Autodesk Inventor part; units mm, degrees
ref_plane "YZ Plane" through (0, 0, 0) normal (1, 0, 0) x (0, 1, 0)
ref_plane "XZ Plane" through (0, 0, 0) normal (0, 1, 0) x (-1, 0, 0)
ref_plane "XY Plane" through (0, 0, 0) normal (0, 0, 1) x (1, 0, 0)
sketch "Sketch1" plane through (0, 0, 0) normal (0, 0, 1) x (1, 0, 0)
  line L0 (-12.7, -12.7) -> (12.7, -12.7)
  line L1 (12.7, -12.7) -> (12.7, 12.7)
  line L2 (12.7, 12.7) -> (-12.7, 12.7)
  line L3 (-12.7, 12.7) -> (-12.7, -12.7)
  line L4 (-12.7, -12.7) -> (12.7, 12.7) construction
  line L5 (12.7, -12.7) -> (-12.7, 12.7) construction
  line L6 (-11.1125, -11.1125) -> (11.1125, -11.1125)
  line L7 (11.1125, -11.1125) -> (11.1125, 11.1125)
  line L8 (11.1125, 11.1125) -> (-11.1125, 11.1125)
  line L9 (-11.1125, 11.1125) -> (-11.1125, -11.1125)
  line L10 (-11.1125, -11.1125) -> (11.1125, 11.1125) construction
  line L11 (11.1125, -11.1125) -> (-11.1125, 11.1125) construction
  point P0 (0, 0)
  dimension "d0" = 25.4
  dimension "d1" = 25.4
  dimension "d2" = 1.5875
extrude "Extrusion1" add sketch "Sketch1" along normal mid plane 609.6
properties part number "1in Box Tube"
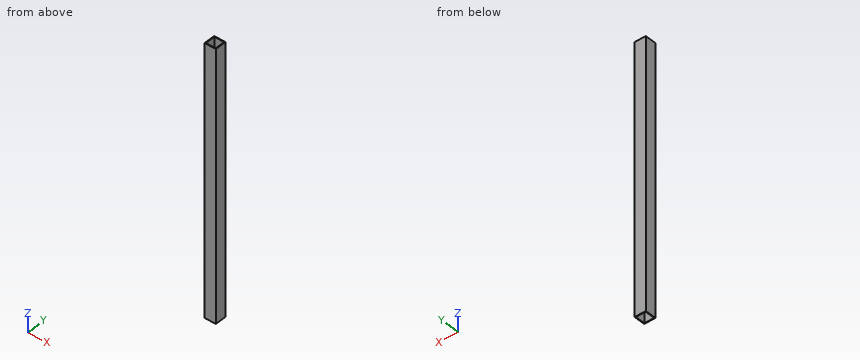
Input: part model. Units: mm. Frame: model coordinates. Coordinates: 2 decimals unless noted, no trailing zeros. Order: outer loops, then holes, each group sorted by start corner. A loop starts at its lowest first (then second) coordinate and runs counter-clockwise, first axis right, second up. Notation, with made-up numbers: M -1,81.5 L 17,81.5 A25 ccw 17,118.5 Z; hole C 14.5,83 d9. An arc over 180 degrees is marked long. Answer as CSV lines item,"result".
1. First-contact query: P1, Ø3, axis at x = -8.5, y = 7, coming from the +Z side. Flat tip, straight axial feed; report the tip coordinate or a pass-through.
Reported:
P1,"through"
2. Material intervals for line 1 (X direction, y = 5, z = 160), sorted ascending. Write a range as from..to.
Reported:
line 1,"-12.7..-11.11, 11.11..12.7"
3. Section B-B (z = -135). Return the cut outline in (x, y).
Reported:
outline,"M -12.7,-12.7 L 12.7,-12.7 L 12.7,12.7 L -12.7,12.7 Z; hole M -11.11,-11.11 L 11.11,-11.11 L 11.11,11.11 L -11.11,11.11 Z"
4. Section A-A (x = 6.75). Return the cut outline in (y, z), then the cut area to 3 significant figures.
Reported:
outline,"M -12.7,-304.8 L -11.11,-304.8 L -11.11,304.8 L -12.7,304.8 Z; M 11.11,-304.8 L 12.7,-304.8 L 12.7,304.8 L 11.11,304.8 Z"
area,"1,940 mm2"
